from build123d import *

# Parameters (mm, degrees)
F1_DEPTH  = 1.5875
F3_DEPTH  = 4.7625
F4_W      = 6.35
F4_H      = 6.35
F5_DEPTH  = 3.175
F6_SIZE   = 1.8598642
F7_W      = 28.575
F7_H      = 3.175
F8_DEPTH  = 1.5875
F9_W      = 25.4
F9_H      = 1.5875
F10_DEPTH = 7.9375
F11_R     = 1.35255
F11_R_2   = 1.8288
F12_DEPTH = 25.4
F13_SIZE  = 1.58749
F14_R     = 0.396875
F15_DEPTH = 7.9375


# Not quite as in the source:
# - a fillet or chamfer is up to 0.001 mm smaller than in the source, because OpenCascade refuses the exact size


with BuildPart() as f1:
    # F0 (on Top) → F1 (new body)
    with BuildSketch(Plane.XY):
        Polygon((-46.7826079092, 22.225), (-127, 22.225), (-127, 17.4625), (-48.7553, 17.4625), (-26.5303, -4.7625), (26.5303, -4.7625), (48.7553, 17.4625), (127, 17.4625), (127, 22.225), (46.7826079092, 22.225), (24.5576079092, 0), (-24.5576079092, 0), align=None)
    extrude(amount=F1_DEPTH)

    # F2 (on face) → F3 (join)
    with BuildSketch(Plane.XY.offset(1.5875)):
        Polygon((-127, 19.05), (-127, 17.4625), (-48.7553, 17.4625), (-26.5303, -4.7625), (26.5303, -4.7625), (48.7553, 17.4625), (127, 17.4625), (127, 19.05), (48.0977359697, 19.05), (25.8727359697, -3.175), (14.2875, -3.175), (14.2875, -1.5875), (-14.2875, -1.5875), (-14.2875, -3.175), (-25.8727359697, -3.175), (-48.0977359697, 19.05), align=None)
    extrude(amount=F3_DEPTH)

    # F4 (on face) → F5 (join, through all)
    with BuildSketch(Plane(origin=(0, 19.05, 0), x_dir=(-1, 0, 0), z_dir=(0, 1, 0))):
        with Locations((-53.5178, 3.175)):
            Rectangle(F4_W, F4_H)
        with Locations((-123.825, 3.175)):
            Rectangle(F4_W, F4_H)
        with Locations((123.825, 3.175)):
            Rectangle(F4_W, F4_H)
        with Locations((53.5178, 3.175)):
            Rectangle(F4_W, F4_H)
    extrude(amount=F5_DEPTH)

    # F6
    f6_edges = [f1.edges().sort_by_distance(p)[0] for p in [
        (-127, 19.84375, 6.35),
        (-120.65, 20.6375, 6.35),
        (-56.6928, 20.6375, 6.35),
        (-50.3428, 20.6375, 6.35),
        (50.3428, 20.6375, 6.35),
        (56.6928, 20.6375, 6.35),
        (120.65, 20.6375, 6.35),
        (127, 19.84375, 6.35),
    ]]
    chamfer(f6_edges, length=F6_SIZE)

    # F7 (on face) → F8 (join)
    with BuildSketch(Plane.XY.offset(6.35)):
        with Locations((0, -3.175)):
            Rectangle(F7_W, F7_H)
    extrude(amount=F8_DEPTH)

    # F9 (on face) → F10 (cut, through all)
    with BuildSketch(Plane.XY.offset(7.9375)):
        with Locations((0, -3.96875)):
            Rectangle(F9_W, F9_H)
    extrude(amount=-F10_DEPTH, mode=Mode.SUBTRACT)

    # F11 (on face) → F12 (cut, through all)
    with BuildSketch(Plane.XZ.offset(3.175)):
        with Locations((53.5178, 3.175)):
            Circle(F11_R)
        with Locations((123.825, 3.175)):
            Circle(F11_R)
        with Locations((-123.825, 3.175)):
            Circle(F11_R)
        with Locations((-53.5178, 3.175)):
            Circle(F11_R)
        with Locations((0, 4.7625)):
            Circle(F11_R_2)
    extrude(amount=-F12_DEPTH, mode=Mode.SUBTRACT)

    # F13 (size 1.5875 in the source; OpenCascade refuses exactly that, so slightly less here)
    f13_edges = [f1.edges().sort_by_distance(p)[0] for p in [
        (-14.2875, -3.96875, 6.35),
        (14.2875, -3.96875, 6.35),
    ]]
    chamfer(f13_edges, length=F13_SIZE)

    # F14 (on face) → F15 (cut, through all)
    with BuildSketch(Plane.XY.offset(7.9375)):
        with Locations((-12.7, -3.175)):
            Circle(F14_R)
        with Locations((12.7, -3.175)):
            Circle(F14_R)
    extrude(amount=-F15_DEPTH, mode=Mode.SUBTRACT)


solid = f1.part
Check sheet for the modelled part. Datum: model origin and axes. Units: mm. A direction names the side the tool comes from. Round coordinates to 2 decimals unless told otherwise and drop trailing zeros. Write each loop counter-clockwise with the first axis right and the second up, starting at its lowest first coordinate (ties: lowest second). Pieces come first, ordered by that corner, then holes. Notation, with made-up numbers: (38, 10) - (97, 10) arc R20 cw to (97, 43) - close; hole circle Ø3 at (25.25, 86.25). An arc over 180 degrees is marked (long way). Return JSON: item names as keys, results as strings.
Q1. Cross-section at B-B (x = 44.5). Record the boundary of the cut face in (y, z), then the cut area to 3 significant figures.
Returned:
{"outline": "(13.21, 0) - (19.94, 0) - (19.94, 1.59) - (15.45, 1.59) - (15.45, 6.35) - (13.21, 6.35) - close", "area": "21.4 mm²"}
Q2. Depth check by flat-ended pin: P1, Ø1.3, axis at y = -4.5, z = 4.5, coming from the -X side; P2, Ø1, axis at y = -3.5, z = 5.5, coming from the -X side; P3, Ø2.5, axis at x = 1, z = 5.5, coming from the -Y side (3 decimals). Enter the tip coordinate at first touch or a pass-through.
Returned:
{"P1": "stops at x = -27.44", "P2": "stops at x = -28.29", "P3": "stops at y = -3.175"}
Q3. Scan lines: L1, parallel to X at y = -2, z = 5; L2, parallel to Y at x = 59, z = 1.5 (1 decimal); L3, parallel to X at y = 14.25, z = 0.75. Record each from-to range of solid material in increasing order. Write a range as from..to.
Returned:
{"L1": "x = -29.29..-27.05, -14.29..-1.81, 1.81..14.29, 27.05..29.29", "L2": "y = 17.5..22.2", "L3": "x = -45.54..-38.81, 38.81..45.54"}
Q4. Access from +Z, -Z, +X, -X, +Y, -Y to the whole of each face (thin tool, end or side, straight path). Record for faces 1 (the flat face through (-88, 17.462, 3)), 2 (the flat face through (35.83, 11.27, 0.78)), 3 (the flat face through (0, -3.175, 2)), 4 (the flat face through (0, -1.588, 7)).
Returned:
{"face 1": "+Z, -Z, -X, -Y", "face 2": "+Z, -Z, +Y", "face 3": "+Z, -Z, -Y", "face 4": "+Z, +Y"}
Q5. Draft check along X on faces 5 (the flat face through (37.14, 8.09, 3.94)), 6 (the flat face through (-90, 22.225, 1)), 7 (the flat face through (37.487, 6.194, 3.131)), 8 (the flat face through (-49, 19.05, 4)). Enter one of: released by +X, released by -X, zero draft, split by the parting line, or undercut.
Returned:
{"face 5": "undercut", "face 6": "zero draft", "face 7": "released by +X", "face 8": "undercut"}
